Build history of the part. All positions in model axes, mm. Face numbers are marked on the shaded views. A direction names the side the tool comes from. Coordinates: 2 decimals unless noted, no trailing zeros. Order: outer loops, then holes, each group sorted by start corner. A loop starts at its lowest first (then second) coordinate and runs counter-clockwise, first axis right, second up. Notation, with made-up numbers: (-11.5, 35.25) - (30.5, 35.25) arc R9 ccw to (30.5, 51.25) - close; hole circle Ø2 at (25, 68.25). An arc over 180 degrees is marked (long way). Return JSON: item names as keys, results as strings.
Autodesk Inventor part; units mm, degrees
ref_plane "YZ Plane" through (0, 0, 0) normal (1, 0, 0) x (0, 1, 0)
ref_plane "XZ Plane" through (0, 0, 0) normal (0, 1, 0) x (-1, 0, 0)
ref_plane "XY Plane" through (0, 0, 0) normal (0, 0, 1) x (1, 0, 0)
sketch "Эскиз4" plane through (0, 0, 0) normal (0, 0, 1) x (1, 0, 0)
  line L0 (0, 0) -> (-20, 0)
  line L1 (-20, 0) -> (-20, 25)
  line L2 (-16, 29) -> (-4, 29)
  line L3 (0, 25) -> (0, 0)
  line L4 (-4, 29) -> (0, 25)
  line L5 (-16, 29) -> (-20, 25)
  point P0 (-20, 29)
  point P1 (0, 29)
  dimension "d14" = 20
  dimension "d15" = 29
  dimension "d16" = 4
  dimension "d17" = 4
  dimension "d18" = 4
  dimension "d19" = 4
revolve "Вращение3" add sketch "Эскиз4" angle 360 about axis through (0, 0, 0) along (-1, 0, 0)
sketch "Эскиз5" plane through (0, 0, 0) normal (1, 0, 0) x (0, 0, -1)
  line L0 (0, 0) -> (0, 20) construction
  dimension "d21" = 20
hole "Отверстие1" at (0, 20, 0) direction (-1, 0, 0) diameter 4 end through all
sketch "Эскиз6" plane through (0, 0, 0) normal (1, 0, 0) x (0, 0, -1)
  point P0 (0, 0)
  point P1 (0, 0)
hole "Отверстие2" at (0, 0, 0) direction (-1, 0, 0) diameter 20 depth 7
properties part number "711122"
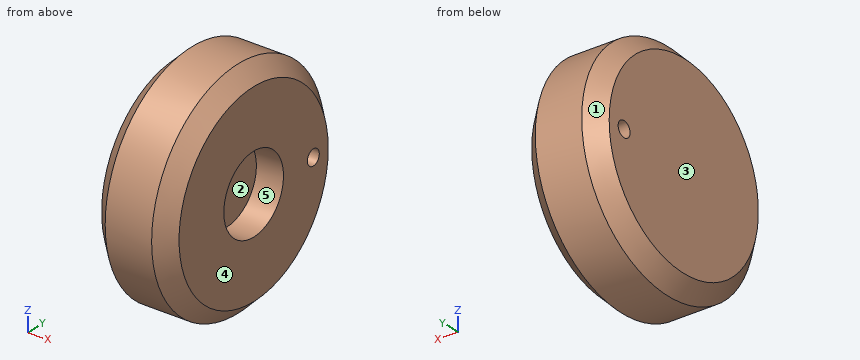
1. Cut at C-C on x = -18. Give the cut face in (y, z).
Check values:
{"outline": "circle Ø54 at (0, 0); hole circle Ø4 at (20, 0)"}
2. Mould opens along Z. For the marked faces 1, 2 and 3 say: pulls with the +Z half, pulls with the -Z half, needs draft (parallel to the pull), parting line crosses it, or undercut.
Check values:
{"face 1": "parting line crosses it", "face 2": "undercut", "face 3": "needs draft"}
3. Cut at A-A on z = 0. Give the cut face in (x, y).
Check values:
{"outline": "(-20, -25) - (-16, -29) - (-4, -29) - (0, -25) - (0, -10) - (-7, -10) - (-7, 10) - (0, 10) - (0, 18) - (-20, 18) - close; (-20, 22) - (0, 22) - (0, 25) - (-4, 29) - (-16, 29) - (-20, 25) - close"}
4. Probe L1, parallel to Y at x = -2.25, z = 0; L2, parallel to Z at x = -4.5, y = 0; L3, parallel to Y at x = -3.25, z = 0. List the from-to ranges inside material, lowest first.
Check values:
{"L1": "-27.25 to -10, 10 to 18, 22 to 27.25", "L2": "-29 to -10, 10 to 29", "L3": "-28.25 to -10, 10 to 18, 22 to 28.25"}
5. Tool access for the marked faces 4 and 5: list every direction of +Z, -Z, +X, -X, +Y, -Y with a clear straight run to the whole face (end or side of a thin tool).
Check values:
{"face 4": "+Z, -Z, +X, +Y, -Y", "face 5": "+X"}
6. Drop flat-ended pins along their axis: pin 1 (3 mm diameter, centred on x = -17.5, y = 10, fed in from -Z); pin 2 (1.5 mm diameter, centred on x = -11.5, z = 12, fed in from -Y); pin 3 (3 mm diameter, centred on x = -9.5, z = -11.5, fed in from -Y). Give the stop position or say it passes through.
Check values:
{"pin 1": "z = -27.31", "pin 2": "y = -26.73", "pin 3": "y = -27.22"}
7. Cut at B-B on y = 0. Give the cut face in (x, z).
Check values:
{"outline": "(-20, -25) - (-16, -29) - (-4, -29) - (0, -25) - (0, -10) - (-7, -10) - (-7, 10) - (0, 10) - (0, 25) - (-4, 29) - (-16, 29) - (-20, 25) - close"}
